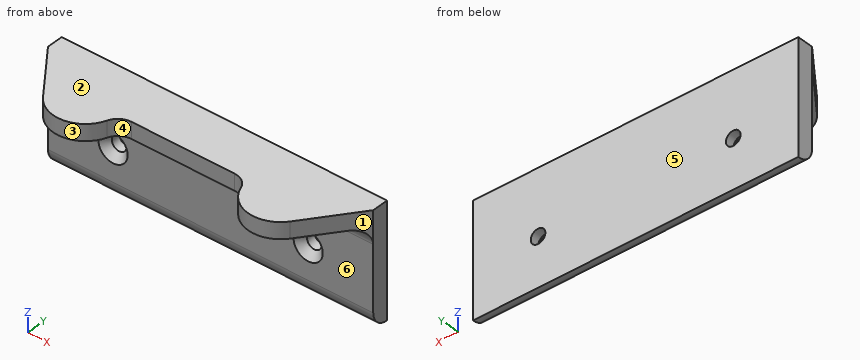
```python
from build123d import *

# Parameters (mm, degrees)
F0_W           = 100
F0_H           = 35
F1_DEPTH       = 5
F3_DEPTH       = 5
F4_R           = 5
F5_R           = 4.99999
F7_D           = 4.5
F7_CSINK_D     = 8.96
F7_CSINK_ANGLE = 90


# Not quite as in the source:
# - a fillet or chamfer is up to 0.001 mm smaller than in the source, because OpenCascade refuses the exact size


with BuildPart() as f1:
    # F0 (on Front) → F1 (new body)
    with BuildSketch(Plane.XZ):
        with Locations((0, 7.5)):
            Rectangle(F0_W, F0_H)
    extrude(amount=F1_DEPTH)

    # F2 (on face) → F3 (join)
    with BuildSketch(Plane.XY.offset(25)):
        with BuildLine():
            Line((-50, -5), (-38, -21))
            ThreePointArc((-38, -21), (-26.8377223398, -24.4868329805), (-20, -15))
            Line((-20, -15), (20, -15))
            ThreePointArc((20, -15), (26.8377223398, -24.4868329805), (38, -21))
            Line((38, -21), (50, -5))
            Line((50, -5), (-50, -5))
        make_face()
    extrude(amount=-F3_DEPTH)

    # F4
    f4_edges = [f1.edges().sort_by_distance(p)[0] for p in [
        (-20, -15, 22.5),
        (0, -5, 20),
        (20, -15, 22.5),
    ]]
    fillet(f4_edges, radius=F4_R)

    # F5 (radius 5 in the source; OpenCascade refuses exactly that, so slightly less here)
    f5_edges = [f1.edges().sort_by_distance(p)[0] for p in [
        (0, -5, -10),
    ]]
    fillet(f5_edges, radius=F5_R)

    # F7 (through all)
    with Locations(Plane.XZ.offset(5)):
        with Locations((-30, 5), (30, 5)):
            CounterSinkHole(F7_D / 2, F7_CSINK_D / 2, counter_sink_angle=F7_CSINK_ANGLE)


solid = f1.part
```
Source: CAD feature listing. Evaluate the final solid. Frame: model axes, mm. Face numbers are marked on the shaded views. A direction names the side the tool comes from. Round coordinates to 2 decimals unless told otherwise and drop trailing zeros. Write each loop counter-clockwise with the first axis right and the second up, starting at its lowest first coordinate (ties: lowest second). Pieces come first, ordered by that corner, then holes. Notation, with made-up numbers: M -19.75,67 L 22.25,67 A16 ccw 22.25,85 Z; hole C 14,9.5 d3. An arc over 180 degrees is marked long. Answer as a JSON object with one key per item and string values. Group by question number.
(1) Reachability of the marked faces 4, 5 and 6 from +Z, -Z, +X, -X, +Y, -Y: full face, straight path, thin tool, end or side. Return the list, or none.
(2) Section query C-C on y = -23.25. Output: boundary loops of the cut face in (x, z).
(3) Mould query, pull axis X, two halves, no side actions, for the marked faces 1, 2 and 3. Classes: +X half, -X half, draft (parallel to the pull), parting line (faces both ways), or undercut.
(4) Ray query, line 1 (X direction, y = -1.25, z = 5); line 2 (Y direction, x = 45.5, z = 13); line 3 (Z direction, x = -30, y = -2.1). Return the intervals inside material, ascending. Write a range as [from, to].
(5) First-contact query: pin 1 (7.5 mm diameter, centred on x = 18.5, y = -15.5, fed in from -Z); pin 2 (10 mm diameter, centred on x = 34.5, z = 0.5, fed in from +Y); pin 3 (4 mm diameter, centred on x = -7, z = 22, fed in from -Y); pin 4 (1.5 mm diameter, centred on x = -10.5, z = 7.5, fed in from -Y). Flat tips, straight axial feed; report the tip coordinate or a pass-through.
(6) Section query B-B on z = 5. Output: boundary loops of the cut face in (x, y).
Computed values:
{
 "1": {"face 4": "+Z, -Z, -Y", "face 5": "+Z, -Z, +X, -X, +Y", "face 6": "-Z, +X, -X, -Y"},
 "2": {"outline": "M -35.65,20 L -24.35,20 L -24.35,25 L -35.65,25 Z; M 24.35,20 L 35.65,20 L 35.65,25 L 24.35,25 Z"},
 "3": {"face 1": "+X half", "face 2": "draft", "face 3": "undercut"},
 "4": {"line 1": "[-50, -32.25], [-27.75, 27.75], [32.25, 50]", "line 2": "[-5, 0]", "line 3": "[-9.54, 2.75], [7.25, 25]"},
 "5": {"pin 1": "z = 20", "pin 2": "y = 0", "pin 3": "y = -15", "pin 4": "y = -5"},
 "6": {"outline": "M -50,-5 L -34.48,-5 L -32.25,-2.77 L -32.25,0 L -50,0 Z; M -27.75,-2.77 L -25.52,-5 L 25.52,-5 L 27.75,-2.77 L 27.75,0 L -27.75,0 Z; M 32.25,-2.77 L 34.48,-5 L 50,-5 L 50,0 L 32.25,0 Z"}
}
